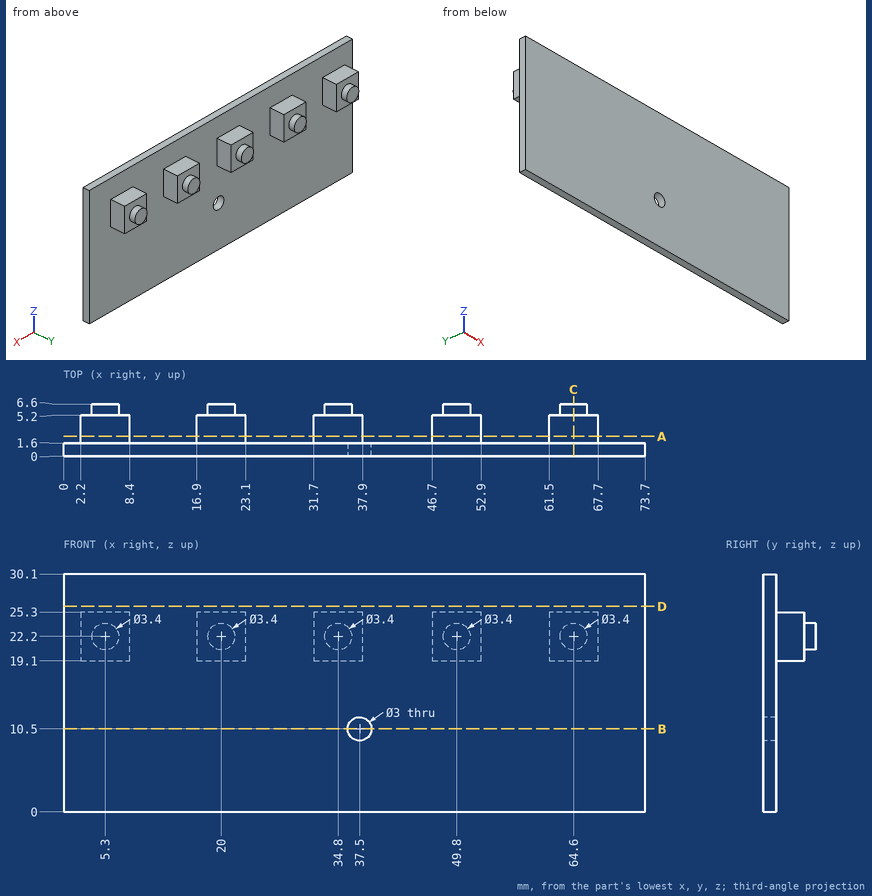
Answer from the drawing. Dimensions are ordinates in mm from the lowest x, y and z of the part. Give positions to 0.01 mm unless a question says otherwise; leave off trailing zeros. Order: outer loops, then holes, each group sorted by start corner. A loop starts at its lowest first (then second) coordinate and runs counter-clockwise, first axis right, second up. Notation, with made-up numbers: (-7.75, -36) - (31.25, -36) arc R28 ccw to (31.25, -15) - close; hole circle Ø6 at (42, 49.5). An arc over 180 degrees is marked (long way). One line per item, written item: value. Start each with the question number.
1) Given pin 1 Ø3 at (x, y) = (4.5, 4) entering from -Z; pin 2 Ø1.1 at (x, y) = (20, 4) entering from +Z; pin 3 Ø1.8 at (y, z) = (4, 21) entering from +X, each flat-ended and moving along its own axis, determine where each tip first touches the part or whether it passes through.
2) A cutting plane is placed at A-A on y = 2.5. Give the vertices of the cut face in (x, z), then the cut area to 3 significant figures.
3) A cutting plane is placed at B-B on z = 10.5. Give the vertices of the cut face in (x, y).
4) A cutting plane is placed at D-D on z = 26. Give the vertices of the cut face in (x, y).
5) Find the intervals of material crossed by L1, parallel to X at y = 5, z = 21; L2, parallel to Z at x = 37.5, y = 1.25; L3, parallel to X at y = 0.75, z = 10.5, in increasing order.
6) A cutting plane is placed at C-C on x = 64.6. Give the vertices of the cut face in (y, z), then the cut area to 3 significant figures.
Answer sheet:
1. pin 1: stops at z = 19.1
1. pin 2: stops at z = 25.3
1. pin 3: stops at x = 67.7
2. outline: (2.2, 19.1) - (8.4, 19.1) - (8.4, 25.3) - (2.2, 25.3) - close; (16.9, 19.1) - (23.1, 19.1) - (23.1, 25.3) - (16.9, 25.3) - close; (31.7, 19.1) - (37.9, 19.1) - (37.9, 25.3) - (31.7, 25.3) - close; (46.7, 19.1) - (52.9, 19.1) - (52.9, 25.3) - (46.7, 25.3) - close; (61.5, 19.1) - (67.7, 19.1) - (67.7, 25.3) - (61.5, 25.3) - close
2. area: 192 mm2
3. outline: (0, 0) - (36, 0) - (36, 1.6) - (0, 1.6) - close; (39, 0) - (73.7, 0) - (73.7, 1.6) - (39, 1.6) - close
4. outline: (0, 0) - (73.7, 0) - (73.7, 1.6) - (0, 1.6) - close
5. L1: x = 2.2 to 8.4, 16.9 to 23.1, 31.7 to 37.9, 46.7 to 52.9, 61.5 to 67.7
5. L2: z = 0 to 9, 12 to 30.1
5. L3: x = 0 to 36, 39 to 73.7
6. outline: (0, 0) - (1.6, 0) - (1.6, 19.1) - (5.2, 19.1) - (5.2, 20.5) - (6.6, 20.5) - (6.6, 23.9) - (5.2, 23.9) - (5.2, 25.3) - (1.6, 25.3) - (1.6, 30.1) - (0, 30.1) - close
6. area: 75.2 mm2
